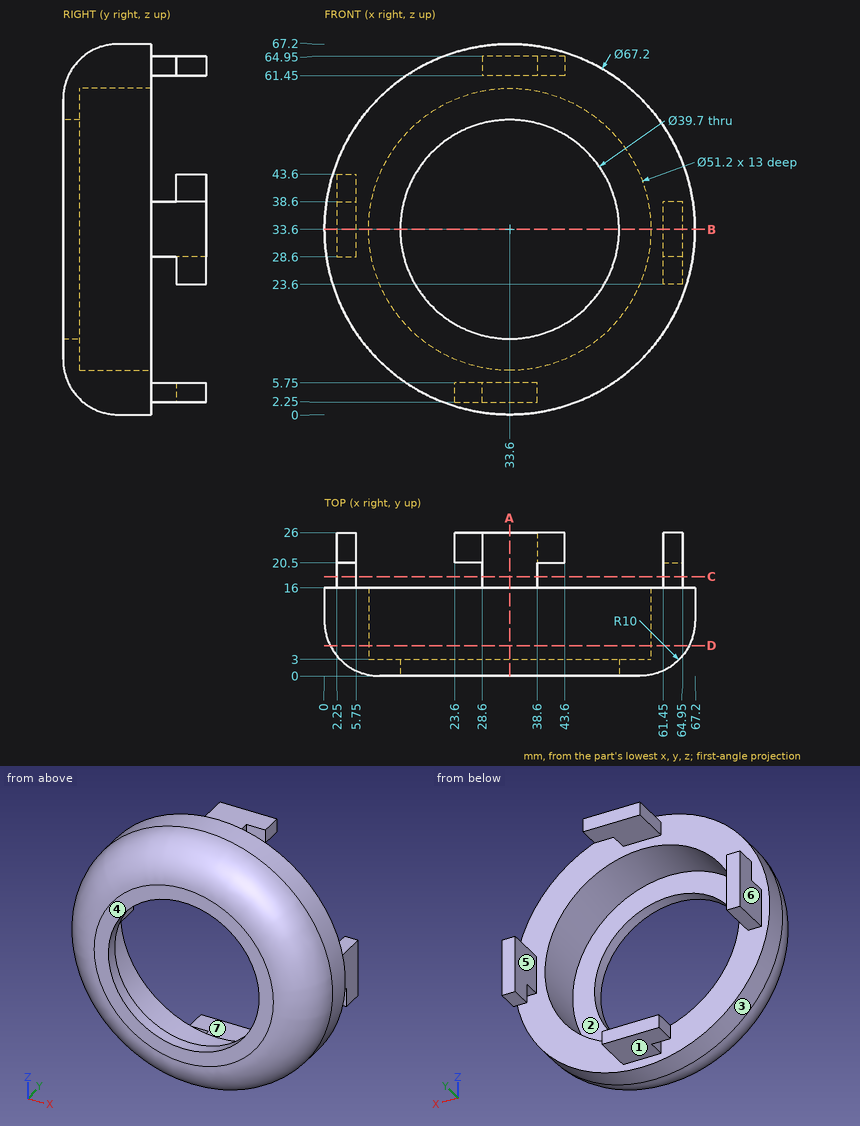
For this review, use the dimensioned drawing (mm, ordinates from the lowest corner) and the shaded views. A direction names the side the tool comes from. Round coordinates to 2 decimals unless told otherwise and drop trailing zeros. Order: outer loops, then holes, each group sorted by start corner. A loop starts at its lowest first (then second) coordinate and runs counter-clockwise, first axis right, second up.
1) Consider section D-D (y = 5.5). State the section outline as (x, z) points.
The answers:
outline: circle Ø65.06 at (33.6, 33.6); hole circle Ø51.2 at (33.6, 33.6)
2) Clearance check with flat-ended pins moving along their axes: pin 1 Ø4 at (x, z) = (4, 41.5) entering from -Y; pin 2 Ø6 at (x, z) = (32, 54.5) entering from +Y; pin 3 Ø5 at (y, z) = (12, 38) entering from -X. State where each tip first meets the part, or that it passes through.
The answers:
pin 1: stops at y = 1.36
pin 2: stops at y = 3
pin 3: stops at x = 0.05
3) Draft analysis for pull direction Z (two halves, no side actions). For the marked faces 1, 2, 3 and 4, state which applies: released by +Z, released by -Z, zero draft, split by the parting line, or undercut.
The answers:
face 1: released by -Z
face 2: undercut
face 3: split by the parting line
face 4: zero draft
4) Consider section B-B (z = 33.6). State the section outline as (x, y) points, plus the area to 3 significant figures.
The answers:
outline: (0, 10) arc R10 ccw to (10, 0) - (13.75, 0) - (13.75, 3) - (8, 3) - (8, 16) - (5.75, 16) - (5.75, 26) - (2.25, 26) - (2.25, 16) - (0, 16) - close; (53.45, 0) - (57.2, 0) arc R10 ccw to (67.2, 10) - (67.2, 16) - (64.95, 16) - (64.95, 26) - (61.45, 26) - (61.45, 16) - (59.2, 16) - (59.2, 3) - (53.45, 3) - close
area: 318 mm2
5) Consider section C-C (y = 18). State the section outline as (x, z) points.
The answers:
outline: (2.25, 28.6) - (5.75, 28.6) - (5.75, 38.6) - (2.25, 38.6) - close; (28.6, 2.25) - (38.6, 2.25) - (38.6, 5.75) - (28.6, 5.75) - close; (28.6, 61.45) - (38.6, 61.45) - (38.6, 64.95) - (28.6, 64.95) - close; (61.45, 28.6) - (64.95, 28.6) - (64.95, 38.6) - (61.45, 38.6) - close
6) Machinability: for the marked faces 5, 6 and 7, which of the approach directions +Z, -Z, +X, -X, +Y, -Y give a long, thin tool a straight path to every point of the face, cutting with its end or side? Answer none if there is none.
The answers:
face 5: +Z, -Z, +Y
face 6: +Z, -Z, -X, +Y
face 7: +X, -X, +Y
7) For L1, parallel to X at y = 9.5, z = 33.6; L2, parallel to X at y = 0.95, z = 33.6; L3, parallel to Y at x = 53.5, z = 21.5, list the stretches that pass through material, from the lowest coordinate up.
The answers:
L1: x = 0.01 to 8, 59.2 to 67.19
L2: x = 5.75 to 13.75, 53.45 to 61.45
L3: y = 0 to 3
8) Consider section A-A (x = 33.6). State the section outline as (y, z) points.
The answers:
outline: (0, 10) arc R10 ccw to (10, 0) - (16, 0) - (16, 2.25) - (26, 2.25) - (26, 5.75) - (16, 5.75) - (16, 8) - (3, 8) - (3, 13.75) - (0, 13.75) - close; (0, 53.45) - (3, 53.45) - (3, 59.2) - (16, 59.2) - (16, 61.45) - (26, 61.45) - (26, 64.95) - (16, 64.95) - (16, 67.2) - (10, 67.2) arc R10 ccw to (0, 57.2) - close
